from build123d import *

# Parameters (mm, degrees)
SKETCH1_R                = 6
SKETCH1_R_2              = 4.75
BOSS_EXTRUDE1_DEPTH      = 13
BOSS_EXTRUDE2_DEPTH      = 14.4
BOSS_EXTRUDE2_DEPTH_BACK = 13
SKETCH2_R                = 4.75
BOSS_EXTRUDE3_START      = -55.5
SKETCH3_R                = 6
BOSS_EXTRUDE3_DEPTH      = 55.5
SKETCH4_R                = 4.75
BOSS_EXTRUDE4_DEPTH      = 85
CHAMFER1_SIZE2           = 10
CHAMFER1_SIZE            = 1.25
CUT_EXTRUDE1_DEPTH       = 15
CUT_EXTRUDE1_DEPTH_BACK  = 15


with BuildPart() as part:
    # Sketch1 → Boss-Extrude1 (new body)
    with BuildSketch(Plane.XY):
        with BuildLine():
            Line((-23.236982917, -5.200252391), (-13.344706072, -2.986439328))
            ThreePointArc((-13.344706072, -2.986439328), (-11.654410969, -1.929360589), (-10.999902799, -0.046242948))
            ThreePointArc((-10.999902799, -0.046242948), (-10.237754277, 4.023479509), (-8.025101164, 7.5231477))
            ThreePointArc((-8.025101164, 7.5231477), (-7.243992277, 9.150122037), (-7.537669453, 10.930832655))
            ThreePointArc((-7.537669453, 10.930832655), (0, 23.2), (7.537669453, 10.930832655))
            ThreePointArc((7.537669453, 10.930832655), (7.243992277, 9.150122037), (8.025101164, 7.5231477))
            ThreePointArc((8.025101164, 7.5231477), (10.237754277, 4.023479509), (10.999902799, -0.046242948))
            ThreePointArc((10.999902799, -0.046242948), (11.654410969, -1.929360589), (13.344706072, -2.986439328))
            Line((13.344706072, -2.986439328), (23.236982917, -5.200252391))
            ThreePointArc((23.236982917, -5.200252391), (25.210855565, -6.682799479), (25.404539286, -9.143816691))
            ThreePointArc((25.404539286, -9.143816691), (0, -27), (-25.404539286, -9.143816691))
            ThreePointArc((-25.404539286, -9.143816691), (-25.210855565, -6.682799479), (-23.236982917, -5.200252391))
        make_face()
        with Locations(Location((0, 0, 0), (0, 0, 180))):
            Circle(SKETCH1_R, mode=Mode.SUBTRACT)
        with Locations(Location((0, 14.75, 0), (0, 0, 180))):
            Circle(SKETCH1_R_2, mode=Mode.SUBTRACT)
    extrude(amount=BOSS_EXTRUDE1_DEPTH)

    # Sketch2 → Boss-Extrude2 (add, two sides: drawn at the far end of the back side and taken through both)
    with BuildSketch(Plane.XY.offset(13).offset(-BOSS_EXTRUDE2_DEPTH_BACK)):
        with Locations((0, 14.75)):
            Circle(SKETCH2_R)
    extrude(amount=BOSS_EXTRUDE2_DEPTH + BOSS_EXTRUDE2_DEPTH_BACK)

    # Sketch3 → Boss-Extrude3 (add)
    with BuildSketch(Plane.XY.offset(13).offset(BOSS_EXTRUDE3_START)):
        Circle(SKETCH3_R)
    extrude(amount=BOSS_EXTRUDE3_DEPTH)

    # Sketch4 → Boss-Extrude4 (add)
    with BuildSketch(Plane(origin=(0, 0, -42.5), x_dir=(-1, 0, 0), z_dir=(0, 0, -1))):
        Circle(SKETCH4_R)
    extrude(amount=BOSS_EXTRUDE4_DEPTH)

    # Chamfer1
    chamfer1_edges = [part.edges().sort_by_distance(p)[0] for p in [
        (4.75, 0, -42.5),
    ]]
    chamfer1_side = [part.faces().sort_by_distance(p)[0] for p in [
        (4.775, 0, -42.5),
    ]]
    chamfer(chamfer1_edges, length=CHAMFER1_SIZE - 0.0001, length2=CHAMFER1_SIZE2 - 0.0001, reference=chamfer1_side[0])  # a hair under: the kernel refuses the full size

    # Sketch5 → Cut-Extrude1 (cut, two sides: drawn at the far end of the back side and taken through both)
    with BuildSketch(Plane(origin=(0, 0, 0), x_dir=(0, 0, -1), z_dir=(1, 0, 0)).offset(-CUT_EXTRUDE1_DEPTH_BACK)):
        with BuildLine():
            Line((127.5, 3.25), (87, 3.25))
            ThreePointArc((87, 3.25), (83.953206786, 4.863584298), (81.962073187, 7.678187319))
            Line((81.962073187, 7.678187319), (127.5, 7.678187319))
            Line((127.5, 7.678187319), (127.5, 4.75))
            Line((127.5, 4.75), (127.5, 3.25))
        make_face()
    extrude(amount=CUT_EXTRUDE1_DEPTH + CUT_EXTRUDE1_DEPTH_BACK, mode=Mode.SUBTRACT)


solid = part.part
Source: CAD feature listing. Evaluate the final solid. Frame: model axes, mm. A direction names the side the tool comes from. Round coordinates to 2 decimals unless told otherwise and drop trailing zeros. Loops run counter-clockwise (first coordinate to the right, second up) from the corner with the lowest first, then second, coordinate; pieces in that order, holes last. Notation, with made-up numbers: (31.5, -16.75) - (69.5, -16.75) arc R19 cw to (69.5, -11.75) - close; hole circle Ø8 at (-2, 62.5). An arc over 180 degrees is marked (long way). Write item = value, one per line. Start each with the question number.
(1) Section query C-C, the plane z = 16.5. Output: boundary loops of the cut face in (x, y), plus the area to 3 significant figures.
(2) Pull-direction query (Y, two-part tool) for faces 6 (the face through (0, -27, 6)), 7 (the face through (18.222, -4.078, 6.409)), 8 (the face through (-7.25, 9.12, 6.41)), 9 (the face through (7.24, 9.18, 6.41)); classes: +Y half, -Y half, draft (parallel to the pull), parting line (faces both ways), or undercut.
(3) Section query D-D, the plane z = -20. Output: boundary loops of the cut face in (x, y).
(4) Pin query (flat end, axial travel): pin 1 (15 mm diameter, centred on x = -9, y = 1, fed in from +Z); pin 2 (5 mm diameter, centred on x = -8.5, y = -18, fed in from -Z); pin 3 (1.5 mm diameter, centred on x = -0.5, z = -0.5, fed in from +Y); pin 4 (3.5 mm diameter, centred on x = -1, z = -116, fed in from +Y). Return the tip coordinate at first contact, or that it passes through.
(5) Section query A-A, the plane y = 14.75. Output: boundary loops of the cut face in (x, z), plus the area to 4 significant figures.
(6) Set-up query: faces 1 (the face through (-6, 0, -22)), 2 (the face through (-0.241, 23.197, 6.409)), 3 (the face through (0, 3.25, -108)), 4 (the face through (4.53, 16.18, 20.1)), 5 (the face through (-18.36, -4.11, 6.41)). Return all of +Z, -Z, +X, -X, +Y, -Y with unobstructed straight access to the full face (end or side cutting, diameter ignored); none if empty.
(7) Ray query, line 1 along Z through (x, y) = (17.5, -20); line 2 along Z through (x, y) = (4.5, 0); line 3 along Y through (x, z) = (-4.5, -24). Return the intervals inside material, ascending. Write a range as from..to.
Conclusion:
q1.outline = circle Ø9.5 at (0, 14.75)
q1.area = 70.9 mm2
q2.face_6 = -Y half
q2.face_7 = +Y half
q2.face_8 = undercut
q2.face_9 = undercut
q3.outline = circle Ø12 at (0, 0)
q4.pin_1 = 13
q4.pin_2 = 0
q4.pin_3 = 23.2
q4.pin_4 = 3.25
q5.outline = (-8.45, 0) - (8.45, 0) - (8.45, 13) - (4.75, 13) - (4.75, 27.4) - (-4.75, 27.4) - (-4.75, 13) - (-8.45, 13) - close
q5.area = 356.5 mm2
q6.face_1 = -Z
q6.face_2 = +Z, -Z
q6.face_3 = -Z, +X, -X, +Y
q6.face_4 = +Z
q6.face_5 = +Z, -Z, -X, +Y
q7.line_1 = 0..13
q7.line_2 = -127.5..13
q7.line_3 = -3.97..3.97
